from build123d import *

# Parameters (mm, degrees)
BOSS_EXTRUDE2_DEPTH   = 100
CUT_EXTRUDE1_DEPTH    = 127.933135767
FILLET1_R             = 20
F_1_0MM_DOWEL_HOLE2_D = 8


with BuildPart() as part:
    # Sketch1 → Boss-Extrude2 (new body)
    with BuildSketch(Plane.XY):
        with BuildLine():
            Line((0, 0), (0, 8))
            Line((0, 8), (25, 8))
            Line((25, 8), (25, 0))
            Line((25, 0), (22.7, 0))
            ThreePointArc((22.7, 0), (20.979270691, -0.542543867), (19.880922138, -1.97393957))
            Line((19.880922138, -1.97393957), (-7, -75.828666157))
            Line((-7, -75.828666157), (-20, -75.828666157))
            Line((-20, -75.828666157), (5.131717491, -3.99064426))
            ThreePointArc((5.131717491, -3.99064426), (4.746623467, -1.263902765), (2.3, 0))
            Line((2.3, 0), (0, 0))
        make_face()
    extrude(amount=-BOSS_EXTRUDE2_DEPTH)

    # Sketch3 → Cut-Extrude1 (cut, through all)
    with BuildSketch(Plane(origin=(5.815996282, -2.03466036, 0), x_dir=(0, 0, 1), z_dir=(-0.9439058304641529, 0.33021475317704674, 0))):
        with BuildLine():
            Line((-90, -7.448753356), (-10, -7.448753356))
            Line((-10, -7.448753356), (-10, -48.179415166))
            ThreePointArc((-10, -48.179415166), (-15.857864376, -62.321550789), (-30, -68.179415166))
            Line((-30, -68.179415166), (-70, -68.179415166))
            ThreePointArc((-70, -68.179415166), (-84.142135624, -62.321550789), (-90, -48.179415166))
            Line((-90, -48.179415166), (-90, -7.448753356))
        make_face()
    extrude(amount=-CUT_EXTRUDE1_DEPTH, mode=Mode.SUBTRACT)

    # Fillet1
    fillet1_edges = [part.edges().sort_by_distance(p)[0] for p in [
        (-13.5, -75.828666157, -100),
        (-13.5, -75.828666157, 0),
    ]]
    fillet(fillet1_edges, radius=FILLET1_R)

    # Ø1.0mm Dowel Hole2 (through all)
    with Locations(Plane(origin=(0, 8, 0), x_dir=(1, 0, 0), z_dir=(0, 1, 0))):
        with Locations((12.52505341, 75.033294682), (12.5, 25), (52.497529088, 47.667377925)):
            Hole(F_1_0MM_DOWEL_HOLE2_D / 2)


solid = part.part
The listing builds one solid part. Answer for the finished solid, in the listing's coordinates (mm). A direction names the side the tool comes from. Round coordinates to 2 decimals unless told otherwise and drop trailing zeros. Order: outer loops, then holes, each group sorted by start corner. A loop starts at its lowest first (then second) coordinate and runs counter-clockwise, first axis right, second up. Notation, with made-up numbers: (-38, 17.25) -> (8, 17.25) arc R32 ccw to (8, 48.25) -> close; hole circle Ø7 at (63, 66). An arc over 180 degrees is marked (long way). One line per item, written item: value.
Item 1: For faces 5 (the flat face through (0, 4, -49)), 6 (the flat face through (24, 0, -49)), 7 (the flat face through (-10.95, -68.4, -49.72)), 8 (the flat face through (1, 0, -49)), 9 (the cylindrical face through (-10, -69.81, -94.3)), determine the directions among +Z, -Z, +X, -X, +Y, -Y from which every point of the face is accessible in a straight line to the end or side of a thin tool.
Taken from the geometry:
face 5: +Z, -Z, -X, +Y
face 6: +Z, -Z, +X, -Y
face 7: +X, +Y
face 8: +Z, -Z, -X
face 9: -Z, +X, -X, -Y
Item 2: Find section A-A, the plane z = -46. Give the vertices of the cut face in (x, y).
Taken from the geometry:
outline: (-20, -75.83) -> (-7, -75.83) -> (-5.05, -70.47) -> (-16.7, -66.39) -> close; (0, 0) -> (2.3, 0) arc R3 cw to (5.13, -3.99) -> (3.36, -9.07) -> (15.72, -13.39) -> (19.88, -1.97) arc R3 cw to (22.7, 0) -> (25, 0) -> (25, 8) -> (0, 8) -> close
Item 3: Find section D-D, the plane z = -25. Give the vertices of the cut face in (x, y), then the cut area to 3 significant figures.
Taken from the geometry:
outline: (-20, -75.83) -> (-7, -75.83) -> (-4.83, -69.87) -> (-16.49, -65.79) -> close; (0, 0) -> (2.3, 0) arc R3 cw to (5.13, -3.99) -> (3.36, -9.07) -> (8.5, -10.87) -> (8.5, 8) -> (0, 8) -> close; (16.5, -11.26) -> (19.88, -1.97) arc R3 cw to (22.7, 0) -> (25, 0) -> (25, 8) -> (16.5, 8) -> close
area: 305 mm2
Item 4: Find section B-B, the plane y = -44. Give the vertices of the cut face in (x, z).
Taken from the geometry:
outline: (-8.87, -100) -> (4.58, -100) -> (4.58, -90) -> (-8.87, -90) -> close; (-8.87, -10) -> (4.58, -10) -> (4.58, 0) -> (-8.87, 0) -> close
Item 5: Straight lines are drawn through the part: L1, parallel to Z at x = 12.5, y = -5.5; L2, parallel to X at y = 3, z = -25; L3, parallel to Z at x = 12, y = -7. For each, find the intervals that lie inside material, in ascending order.
Taken from the geometry:
L1: z = -100 to -79.03, -71.03 to -29, -21 to 0
L2: x = 0 to 8.5, 16.5 to 25
L3: z = -100 to -79, -71.07 to -28.97, -21.03 to 0
Item 6: Given P1, Ø6.5, axis at y = 4.5, z = -69, coming from the -X side; P2, Ø2.5, axis at x = 1, z = -42, coming from the -Y side; P3, Ø12, axis at x = -4, y = -18, coming from the +Z side; P4, Ø9, axis at x = 12.5, z = -25, coming from the -Y side, each flat-ended and moving along its own axis, determine where each tip first touches the part or whether it passes through.
Taken from the geometry:
P1: stops at x = 0
P2: stops at y = 0
P3: stops at z = 0
P4: stops at y = -13.39
Item 7: Find section C-C, the plane x = 11.5. Give the vertices of the cut face in (y, z).
Taken from the geometry:
outline: (-25, -100) -> (8, -100) -> (8, -78.9) -> (-11.91, -78.9) -> (-11.91, -90) -> (-25, -90) -> close; (-25, -10) -> (-11.91, -10) -> (-11.91, -21.13) -> (8, -21.13) -> (8, 0) -> (-25, 0) -> close; (-11.91, -71.17) -> (8, -71.17) -> (8, -28.87) -> (-11.91, -28.87) -> close
Item 8: For a pull along X with two mould halves and no side action, classify faces 1 (the cylindrical face through (16.52, -2.85, -75.21)), 2 (the cylindrical face through (16.496, -2.846, -25.176)), 3 (the flat face through (9.454, -11.199, -50.56)), 4 (the flat face through (12, 8, -49)) as released by +X, released by -X, zero draft, split by the parting line, or undercut.
Taken from the geometry:
face 1: undercut
face 2: undercut
face 3: released by -X
face 4: zero draft
